CAD build for the part. Positions are in the model's coordinates, mm. A direction names the side the tool comes from. Round coordinates to 2 decimals unless told otherwise and drop trailing zeros. Write each loop counter-clockwise with the first axis right and the second up, starting at its lowest first coordinate (ties: lowest second). Pieces come first, ordered by that corner, then holes. Notation, with made-up numbers: (62, -21.5) -> (104, -21.5) arc R12 ccw to (104, -16.5) -> close; hole circle Ø9 at (6.5, -25). An arc over 180 degrees is marked (long way). Answer in a Markdown table with one row per item. Add a question column.
```python
from build123d import *

# Parameters (mm, degrees)
SKETCH1_W           = 30.48
SKETCH1_H           = 57.15
SKETCH1_R           = 4.7625
SKETCH1_W_2         = 1.5748
SKETCH1_H_2         = 2.5781
BOSS_EXTRUDE1_DEPTH = 6.35
CHAMFER1_SIZE       = 6.35


with BuildPart() as part:
    # Sketch1 → Boss-Extrude1 (new body)
    with BuildSketch(Plane.XY):
        with Locations((0, 28.575)):
            Rectangle(SKETCH1_W, SKETCH1_H)
        with Locations((0, 44.45)):
            Circle(SKETCH1_R, mode=Mode.SUBTRACT)
        with Locations((-11.2014, 44.45)):
            Rectangle(SKETCH1_W_2, SKETCH1_H_2, mode=Mode.SUBTRACT)
        with Locations((11.2014, 44.45)):
            Rectangle(SKETCH1_W_2, SKETCH1_H_2, mode=Mode.SUBTRACT)
    extrude(amount=BOSS_EXTRUDE1_DEPTH)

    # Chamfer1
    chamfer1_edges = [part.edges().sort_by_distance(p)[0] for p in [
        (15.24, 57.15, 3.175),
        (-15.24, 57.15, 3.175),
    ]]
    chamfer(chamfer1_edges, length=CHAMFER1_SIZE)


solid = part.part
```
Item 1: Tool access for faces 4 (the flat face through (0, 0, 3)), 5 (the flat face through (-11.989, 44, 3)): list every direction of +Z, -Z, +X, -X, +Y, -Y with a clear straight run to the whole face (end or side of a thin tool).
Item 2: Two-plate mould, pull along Y, no slides. Class faces 1 (the flat face through (11, 45.739, 3)), 2 (the flat face through (-12.02, 54.02, 3.13)), 3 (the flat face through (0, 29, 0)): +Y half, -Y half, draft (parallel to the pull), parting line (faces both ways), or undercut.
Item 3: Saw through at C-C on x = 0. Give the cut face in (y, z), then the cut area to 3 significant figures.
Item 4: Drill centre lines: probe 1 along Y at (x, z) = (0, 5.25); probe 2 along Y at (x, z) = (-3, 0.5); probe 3 along Y at (x, z) = (9, 3.5). Where is each one in solid material? Low to high.
Item 5: Saw through at B-B on z = 2. Count the separate pieces of the cut face and the enclosed holes in it, then the cut area to 3 significant figures.
Item 6: Pin check, flat tips, straight feed: pin 1 (1.7 mm diameter, centred on x = -11, z = 3.5, fed in from +Y); pin 2 (1.3 mm diameter, centred on x = 11, z = 4, fed in from -Y); pin 3 (8.5 mm diameter, centred on x = 0, y = 44.45, fed in from -Z); pin 4 (1.3 mm diameter, centred on x = 11.5, z = 4.5, fed in from +Y). Stop position of each tip, or through.
Item 7: Saw through at A-A on y = 44.45. Give the cut face in (x, z), then the cut area to 3 significant figures.
Recorded:
| question | item | result |
|---|---|---|
| 1 | face 4 | +Z, -Z, +X, -X, -Y |
| 1 | face 5 | +Z, -Z |
| 2 | face 1 | undercut |
| 2 | face 2 | +Y half |
| 2 | face 3 | draft |
| 3 | outline | (0, 0) -> (39.69, 0) -> (39.69, 6.35) -> (0, 6.35) -> close; (49.21, 0) -> (57.15, 0) -> (57.15, 6.35) -> (49.21, 6.35) -> close |
| 3 | area | 302 mm2 |
| 4 | probe 1 | 0 to 39.69, 49.21 to 57.15 |
| 4 | probe 2 | 0 to 40.75, 48.15 to 57.15 |
| 4 | probe 3 | 0 to 57.04 |
| 5 | separate pieces | 1 |
| 5 | enclosed holes | 3 |
| 5 | area | 1,620 mm2 |
| 6 | pin 1 | y = 55.89 |
| 6 | pin 2 | y = 0 |
| 6 | pin 3 | through |
| 6 | pin 4 | y = 55.19 |
| 7 | outline | (-15.24, 0) -> (-11.99, 0) -> (-11.99, 6.35) -> (-15.24, 6.35) -> close; (-10.41, 0) -> (-4.76, 0) -> (-4.76, 6.35) -> (-10.41, 6.35) -> close; (4.76, 0) -> (10.41, 0) -> (10.41, 6.35) -> (4.76, 6.35) -> close; (11.99, 0) -> (15.24, 0) -> (15.24, 6.35) -> (11.99, 6.35) -> close |
| 7 | area | 113 mm2 |
